Source: CAD feature listing. Evaluate the final solid. Frame: model axes, mm. Face numbers are marked on the shaded views. Give positions to 0.01 mm unless a question says otherwise; leave off trailing zeros. Order: outer loops, then holes, each group sorted by start corner. A loop starts at its lowest first (then second) coordinate and runs counter-clockwise, first axis right, second up. Notation, with made-up numbers: (58, -30.75) - (65, -30.75) arc R30 ccw to (65, -2.75) - close; hole circle Ø3 at (87.5, 65.25). An arc over 180 degrees is marked (long way). One line per item, written item: value. Start each with the question number.
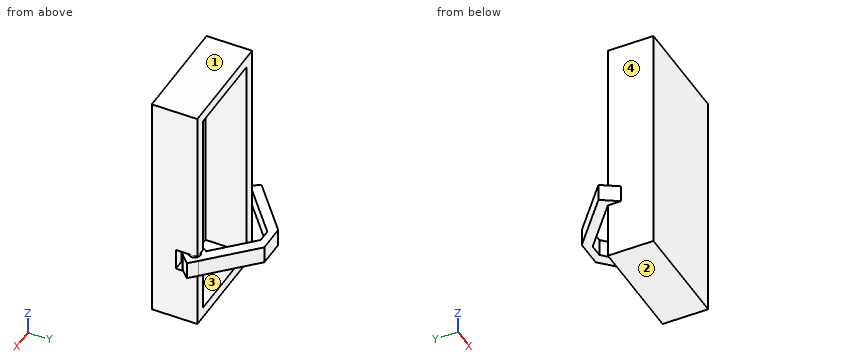
from build123d import *

# Parameters (mm, degrees)
F0_W      = 50.8
F0_H      = 2.54
F1_DEPTH  = 127
F2_W      = 63.5
F2_H      = 26.924
F3_DEPTH  = 6.35
F4_W      = 63.5
F4_H      = 26.924
F5_DEPTH  = 6.35
F6_W      = 12.7
F6_H      = 12.7
F7_DEPTH  = 6.35
F8_R      = 3.175
F9_DEPTH  = 12.7
F11_START = 1.27
F10_W     = 2.54
F10_H     = 2.54
F11_DEPTH = 10.16


with BuildPart() as f1:
    # F0 (on Top) → F1 (new body)
    with BuildSketch(Plane.XY):
        with Locations((0.755213508, -18.3883576206)):
            Rectangle(F0_W, F0_H)
        Polygon((-24.644786492, -19.6583576206), (-24.644786492, -17.1183576206), (-24.644786492, 7.2656423794), (-30.994786492, 7.2656423794), (-30.994786492, -19.6583576206), align=None)
        Polygon((26.155213508, 7.2656423794), (26.155213508, -17.1183576206), (26.155213508, -19.6583576206), (32.505213508, -19.6583576206), (32.505213508, 7.2656423794), align=None)
    extrude(amount=F1_DEPTH)

    # F2 (on face) → F3 (join)
    with BuildSketch(Plane(origin=(0, 0, 0), x_dir=(1, 0, 0), z_dir=(0, 0, -1))):
        with Locations((0.755213508, 6.1963576206)):
            Rectangle(F2_W, F2_H)
    extrude(amount=F3_DEPTH)

    # F4 (on face) → F5 (join)
    with BuildSketch(Plane.XY.offset(127)):
        with Locations((0.755213508, -6.1963576206)):
            Rectangle(F4_W, F4_H)
    extrude(amount=F5_DEPTH)

    # F6 (on face) → F7 (cut, through all)
    with BuildSketch(Plane.YZ.offset(32.505213508)):
        with Locations((0.9156423794, 33.02)):
            Rectangle(F6_W, F6_H)
    extrude(amount=-F7_DEPTH, mode=Mode.SUBTRACT)

    # F8 (on face) → F9 (join, through all)
    with BuildSketch(Plane.XY.offset(26.67)):
        with Locations((29.330213508, 4.0906423794)):
            Circle(F8_R)
    extrude(amount=F9_DEPTH)

    # F10 (on face) → F11 (join)
    with BuildSketch(Plane.XY.offset(26.67).offset(F11_START)):
        with BuildLine():
            ThreePointArc((26.9953469165, 6.4255089708), (30.5938342017, 7.1412925957), (32.632213508, 4.0906423794))
            ThreePointArc((32.632213508, 4.0906423794), (32.3808637244, 2.8270216857), (31.6650800995, 1.7557757879))
            Line((31.6650800995, 1.7557757879), (33.8203415686, -0.3994856812))
            ThreePointArc((33.8203415686, -0.3994856812), (35.1968485395, 1.6606025838), (35.680213508, 4.0906423794))
            ThreePointArc((35.680213508, 4.0906423794), (35.1968485273, 6.5206822043), (33.8203415234, 8.580770485))
            ThreePointArc((33.8203415234, 8.580770485), (29.3302134761, 10.4406423794), (24.8400854475, 8.5807704399))
            Line((24.8400854475, 8.5807704399), (26.9953469165, 6.4255089708))
        make_face()
        with BuildLine():
            ThreePointArc((31.6650800995, 1.7557757879), (26.9953469165, 1.7557757879), (26.9953469165, 6.4255089708))
            Line((26.9953469165, 6.4255089708), (24.8400854475, 8.5807704399))
            ThreePointArc((24.8400854475, 8.5807704399), (24.8400854475, -0.3994856812), (33.8203415686, -0.3994856812))
            Line((33.8203415686, -0.3994856812), (31.6650800995, 1.7557757879))
        make_face()
        with BuildLine():
            Line((3.539213508, 29.8816423794), (24.8400854475, 8.5807704399))
            ThreePointArc((24.8400854475, 8.5807704399), (29.3302134761, 10.4406423794), (33.8203415234, 8.580770485))
            Line((33.8203415234, 8.580770485), (8.0293415685, 34.3717704399))
            Line((8.0293415685, 34.3717704399), (8.0293415685, 29.8816423794))
            Line((8.0293415685, 29.8816423794), (3.539213508, 29.8816423794))
        make_face()
        with BuildLine():
            ThreePointArc((35.680213508, 4.0906423794), (35.1968485395, 1.6606025838), (33.8203415686, -0.3994856812))
            Line((33.8203415686, -0.3994856812), (38.3104696291, 4.0906423794))
            Line((38.3104696291, 4.0906423794), (33.8203415234, 8.580770485))
            ThreePointArc((33.8203415234, 8.580770485), (35.1968485273, 6.5206822043), (35.680213508, 4.0906423794))
        make_face()
        Polygon((-4.2345756454, 29.8816423794), (3.539213508, 29.8816423794), (8.0293415685, 34.3717704399), (-8.0293415685, 34.3717704399), align=None)
        Polygon((8.0293415685, 34.3717704399), (3.539213508, 29.8816423794), (8.0293415685, 29.8816423794), align=None)
        Polygon((-30.994786492, 7.2656423794), (-4.2345756454, 29.8816423794), (-8.0293415685, 29.8816423794), (-8.0293415685, 34.3717704399), (-37.344786492, 9.5962518093), (-33.5500205688, 5.1061237488), align=None)
        Polygon((-8.0293415685, 29.8816423794), (-4.2345756454, 29.8816423794), (-8.0293415685, 34.3717704399), align=None)
        Polygon((-30.994786492, 2.1856423794), (-30.994786492, 7.2656423794), (-33.5500205688, 5.1061237488), (-37.344786492, 9.5962518093), (-30.994786492, -0.3543576206), align=None)
        with Locations((-29.724786492, 0.9156423794)):
            Rectangle(F10_W, F10_H)
    extrude(amount=F11_DEPTH)


solid = f1.part
1. Section D-D on y = -4. Return the cut outline in (x, z), then the cut area to 3 significant figures.
2. Contact query for flat-ended pins moving along their axis: pin 1 Ø4 at (y, z) = (-6.5, 86.5) entering from -X; pin 2 Ø1.5 at (y, z) = (-10, 103) entering from +X; pin 3 Ø5 at (x, z) = (29.5, 30.5) entering from +Y; pin 4 Ø12 at (y, z) = (19, 56.5) entering from +X. Output: stop coordinate, or through.
3. Section B-B on x = 0. Return the cut outline in (y, z), then the cut area to 3 significant figures.
4. Section C-C on z = 64.5. Return the cut outline in (x, y), then the cut area to 3 significant figures.
5. Section A-A on y = -11.5. Return the cut outline in (x, z), then the cut area to 3 significant figures.
6. Ray query, L1, parallel to Z at x = -14, y = -12; L2, parallel to X at y = -15, z = 109.5; L3, parallel to Y at x = -27.5, z = 24. Return the intervals inside material, ascending.
7. Draft query along Z for the marked faces 1, 2, 3 and 4. Return one class per face: pulls with the +Z half, pulls with the -Z half, needs draft (parallel to the pull), parting line crosses it, or undercut.
Data:
1. outline: (-30.99, -6.35) - (32.51, -6.35) - (32.51, 26.67) - (26.16, 26.67) - (26.16, 0) - (-24.64, 0) - (-24.64, 127) - (26.16, 127) - (26.16, 39.37) - (32.51, 39.37) - (32.51, 133.35) - (-30.99, 133.35) - close
1. area: 2,340 mm2
2. pin 1: stops at x = -30.99
2. pin 2: stops at x = 32.51
2. pin 3: stops at y = 15.4
2. pin 4: passes through
3. outline: (-19.66, -6.35) - (7.27, -6.35) - (7.27, 0) - (-17.12, 0) - (-17.12, 127) - (7.27, 127) - (7.27, 133.35) - (-19.66, 133.35) - close; (29.88, 27.94) - (34.37, 27.94) - (34.37, 38.1) - (29.88, 38.1) - close
3. area: 710 mm2
4. outline: (-30.99, -19.66) - (32.51, -19.66) - (32.51, 7.27) - (26.16, 7.27) - (26.16, -17.12) - (-24.64, -17.12) - (-24.64, 7.27) - (-30.99, 7.27) - close
4. area: 471 mm2
5. outline: (-30.99, -6.35) - (32.51, -6.35) - (32.51, 133.35) - (-30.99, 133.35) - close; hole (-24.64, 0) - (26.16, 0) - (26.16, 127) - (-24.64, 127) - close
5. area: 2,420 mm2
6. L1: z = -6.35 to 0, 127 to 133.35
6. L2: x = -30.99 to -24.64, 26.16 to 32.51
6. L3: y = -19.66 to 7.27
7. face 1: pulls with the +Z half
7. face 2: pulls with the -Z half
7. face 3: undercut
7. face 4: needs draft
